The listing builds one solid part. Answer for the finished solid, in the listing's coordinates (mm). A direction names the side the tool comes from. Coordinates: 2 decimals unless noted, no trailing zeros. Order: outer loops, then holes, each group sorted by start corner. A loop starts at its lowest first (then second) coordinate and runs counter-clockwise, first axis right, second up. Notation, with made-up numbers: (3, 41) -> (41, 41) arc R24 cw to (41, 59) -> close; hole circle Ø2 at (12.5, 19.25). An arc over 180 degrees is marked (long way). Return JSON: item names as keys, results as strings.
```python
from build123d import *

# Parameters (mm, degrees)
SKETCH1_W           = 28
SKETCH1_H           = 5
BOSS_EXTRUDE1_DEPTH = 20
CHAMFER1_SIZE       = 15
BOSS_EXTRUDE2_DEPTH = 28
SKETCH3_W           = 3
SKETCH3_H           = 9
CUT_EXTRUDE1_DEPTH  = 12.8
CHAMFER2_SIZE       = 1
FILLET1_R           = 2
CHAMFER3_SIZE       = 0.5
CUT_EXTRUDE2_DEPTH  = 12.8
CHAMFER4_SIZE       = 3
CHAMFER5_SIZE       = 3
SKETCH8_W           = 3.20799886
SKETCH8_H           = 3.210000155
SKETCH8_W_2         = 3.209995615
SKETCH8_H_2         = 3.268000248
CUT_EXTRUDE3_DEPTH  = 5.4
SKETCH9_W           = 136.063633216
SKETCH9_H           = 34.178471192
CUT_EXTRUDE4_DEPTH  = 8
SKETCH10_W          = 4.648757297
SKETCH10_H          = 6.5
BOSS_EXTRUDE3_DEPTH = 10
SKETCH12_W          = 15
SKETCH12_H          = 15
BOSS_EXTRUDE4_DEPTH = 3
SKETCH13_R          = 1.5
CUT_EXTRUDE5_DEPTH  = 5
FILLET2_R           = 3
CHAMFER6_SIZE       = 3


with BuildPart() as part:
    # Sketch1 → Boss-Extrude1 (new body)
    with BuildSketch(Plane(origin=(0, 0, 0), x_dir=(1, 0, 0), z_dir=(0, 1, 0))):
        with Locations((14, 2.5)):
            Rectangle(SKETCH1_W, SKETCH1_H)
    extrude(amount=BOSS_EXTRUDE1_DEPTH)

    # Chamfer1
    chamfer1_edges = [part.edges().sort_by_distance(p)[0] for p in [
        (28, 0, -2.5),
    ]]
    chamfer(chamfer1_edges, length=CHAMFER1_SIZE)

    # Sketch2 → Boss-Extrude2 (add)
    with BuildSketch(Plane.XY):
        Polygon((9.648757297, 6.5), (5, 6.5), (5, 2), (5, 0), (9.648757297, 0), align=None)
    extrude(amount=BOSS_EXTRUDE2_DEPTH)

    # Sketch3 → Cut-Extrude1 (cut)
    with BuildSketch(Plane.XZ):
        with Locations((6.5, 18)):
            Rectangle(SKETCH3_W, SKETCH3_H)
    extrude(amount=-CUT_EXTRUDE1_DEPTH, mode=Mode.SUBTRACT)

    # Chamfer2
    chamfer2_edges = [part.edges().sort_by_distance(p)[0] for p in [
        (8, 3.25, 22.5),
        (8, 3.25, 13.5),
    ]]
    chamfer(chamfer2_edges, length=CHAMFER2_SIZE)

    # Fillet1
    fillet1_edges = [part.edges().sort_by_distance(p)[0] for p in [
        (7.324378649, 6.5, 28),
        (7.324378649, 0, 28),
    ]]
    fillet(fillet1_edges, radius=FILLET1_R)

    # Chamfer3
    chamfer3_edges = [part.edges().sort_by_distance(p)[0] for p in [
        (5, 3.25, 13.5),
        (5, 3.25, 22.5),
    ]]
    chamfer(chamfer3_edges, length=CHAMFER3_SIZE)

    # Sketch4 → Cut-Extrude2 (cut)
    with BuildSketch(Plane.ZY.offset(-5)):
        with BuildLine():
            ThreePointArc((25.5, 1.45), (27.05, 3), (25.5, 4.55))
            ThreePointArc((25.5, 4.55), (23.95, 3), (25.5, 1.45))
        make_face()
        with BuildLine():
            ThreePointArc((10.5, 4.55), (8.95, 3), (10.5, 1.45))
            ThreePointArc((10.5, 1.45), (12.05, 3), (10.5, 4.55))
        make_face()
    extrude(amount=-CUT_EXTRUDE2_DEPTH, mode=Mode.SUBTRACT)

    # Chamfer4
    chamfer4_edges = [part.edges().sort_by_distance(p)[0] for p in [
        (5, 3.25, 0),
        (9.648757297, 3.25, 0),
    ]]
    chamfer(chamfer4_edges, length=CHAMFER4_SIZE)

    # Chamfer5
    chamfer5_edges = [part.edges().sort_by_distance(p)[0] for p in [
        (7.324378649, 6.5, 0),
    ]]
    chamfer(chamfer5_edges, length=CHAMFER5_SIZE)

    # Sketch8 → Cut-Extrude3 (cut)
    # profile 1 of 4: a face of its own
    with BuildSketch(Plane(origin=(0, 20, 0), x_dir=(1, 0, 0), z_dir=(0, 1, 0))):
        with Locations((5.668003112, 2.226999903)):
            Rectangle(SKETCH8_W, SKETCH8_H)
        Polygon((7.122002542, 3.68199998), (6.328001618, 3.68199998), (4.214003682, 3.68199998), (4.214003682, 2.801999915), (4.214003682, 2.091999864), (4.214003682, 0.771999825), (4.858002067, 0.771999825), (6.60200417, 0.771999825), (7.122002542, 0.771999825), (7.122002542, 3.48399987), align=None, mode=Mode.SUBTRACT)
    # profile 2 of 4: a face of its own
    with BuildSketch(Plane(origin=(0, 20, 0), x_dir=(1, 0, 0), z_dir=(0, 1, 0))):
        Polygon((7.122002542, 3.68199998), (7.122002542, 3.48399987), (7.122002542, 0.771999825), (6.60200417, 0.771999825), (4.858002067, 0.771999825), (4.214003682, 0.771999825), (4.214003682, 2.091999864), (4.214003682, 2.801999915), (4.214003682, 3.68199998), (6.328001618, 3.68199998), align=None)
    # profile 3 of 4: a face of its own
    with BuildSketch(Plane(origin=(0, 20, 0), x_dir=(1, 0, 0), z_dir=(0, 1, 0))):
        with Locations((23.709002883, 2.229999751)):
            Rectangle(SKETCH8_W_2, SKETCH8_H_2)
        Polygon((22.254005075, 1.15799997), (22.254005075, 1.283999765), (22.254005075, 3.713999875), (25.16400069, 3.713999875), (25.16400069, 0.749999657), (25.16400069, 0.745999627), (24.429999292, 0.745999627), (22.254005075, 0.745999627), align=None, mode=Mode.SUBTRACT)
    # profile 4 of 4: a face of its own
    with BuildSketch(Plane(origin=(0, 20, 0), x_dir=(1, 0, 0), z_dir=(0, 1, 0))):
        Polygon((22.254005075, 3.713999875), (22.254005075, 1.283999765), (22.254005075, 1.15799997), (22.254005075, 0.745999627), (24.429999292, 0.745999627), (25.16400069, 0.745999627), (25.16400069, 0.749999657), (25.16400069, 3.713999875), align=None)
    extrude(amount=-CUT_EXTRUDE3_DEPTH, mode=Mode.SUBTRACT)

    # Sketch9 → Cut-Extrude4 (cut)
    with BuildSketch(Plane(origin=(0, 0, -5), x_dir=(-1, 0, 0), z_dir=(0, 0, -1))):
        with Locations((-4.69867378, 12.292617934)):
            Rectangle(SKETCH9_W, SKETCH9_H)
    extrude(amount=-CUT_EXTRUDE4_DEPTH, mode=Mode.SUBTRACT)

    # Sketch10 → Boss-Extrude3 (add)
    with BuildSketch(Plane(origin=(0, 0, 3), x_dir=(-1, 0, 0), z_dir=(0, 0, -1))):
        with Locations((-7.324378649, 3.25)):
            Rectangle(SKETCH10_W, SKETCH10_H)
    extrude(amount=BOSS_EXTRUDE3_DEPTH)

    # Sketch12 → Boss-Extrude4 (add)
    with BuildSketch(Plane(origin=(0, 0, -7), x_dir=(-1, 0, 0), z_dir=(0, 0, -1))):
        with Locations((-12.5, 7.5)):
            Rectangle(SKETCH12_W, SKETCH12_H)
    extrude(amount=-BOSS_EXTRUDE4_DEPTH)

    # Sketch13 → Cut-Extrude5 (cut)
    with BuildSketch(Plane.XY.offset(-4)):
        with Locations((17, 3)):
            Circle(SKETCH13_R)
        with Locations((8, 12)):
            Circle(SKETCH13_R)
    extrude(amount=-CUT_EXTRUDE5_DEPTH, mode=Mode.SUBTRACT)

    # Fillet2
    fillet2_edges = [part.edges().sort_by_distance(p)[0] for p in [
        (5, 15, -5.5),
        (20, 0, -5.5),
        (20, 15, -5.5),
    ]]
    fillet(fillet2_edges, radius=FILLET2_R)

    # Chamfer6
    chamfer6_edges = [part.edges().sort_by_distance(p)[0] for p in [
        (9.648757297, 3.25, -4),
    ]]
    chamfer(chamfer6_edges, length=CHAMFER6_SIZE)


solid = part.part
```
Item 1: The part is cut by section A-A on z = 25.5. Determine the outline of the cut face in (x, y).
Answer list:
{"outline": "(5, 0) -> (9.65, 0) -> (9.65, 1.45) -> (5, 1.45) -> close; (5, 4.55) -> (9.65, 4.55) -> (9.65, 6.5) -> (5, 6.5) -> close"}
Item 2: The part is cut by section B-B on y = 3.5. Determine the outline of the cut face in (x, z).
Answer list:
{"outline": "(5, -7) -> (15.59, -7) -> (15.59, -4) -> (12.65, -4) -> (9.65, -1) -> (9.65, 9.03) -> (5, 9.03) -> close; (5, 11.97) -> (9.65, 11.97) -> (9.65, 24.03) -> (5, 24.03) -> (5, 23) -> (5.5, 22.5) -> (7, 22.5) -> (8, 21.5) -> (8, 14.5) -> (7, 13.5) -> (5.5, 13.5) -> (5, 13) -> close; (5, 26.97) -> (9.65, 26.97) -> (9.65, 28) -> (5, 28) -> close; (18.41, -7) -> (20, -7) -> (20, -4) -> (18.41, -4) -> close"}
Item 3: The part is cut by section D-D on y = 13. Determine the outline of the cut face in (x, z).
Answer list:
{"outline": "(5.17, -7) -> (6.88, -7) -> (6.88, -4) -> (5.17, -4) -> close; (9.12, -7) -> (19.83, -7) -> (19.83, -4) -> (9.12, -4) -> close"}
Item 4: Which of the six approach directions +Z, -Z, +X, -X, +Y, -Y give full straight-line access (tool end or side, diameter ignored) to faces 4 (the flat face through (9.649, 3, 14)), 5 (the flat face through (6, 3, 22.5)), 6 (the cylindrical face through (6.8, 11.1, -5.5))?
Answer list:
{"face 4": "+Z, +X, +Y, -Y", "face 5": "-X, +Y, -Y", "face 6": "+Z, -Z"}
Item 5: Flat-ended cylindrical pins translate along their axes: pin 1 (5 mm diameter, centred on x = 13, y = 4.5, fed in from +Z); pin 2 (5 mm diameter, centred on y = 3, z = 25.5, fed in from +X); pin 3 (3 mm diameter, centred on x = 15, y = 10.5, fed in from +Z). Find the tip coordinate at first contact, or state that the pin passes through.
Answer list:
{"pin 1": "z = -1.85", "pin 2": "x = 9.65", "pin 3": "z = -4"}
Item 6: Find the intervals of material crossed by probe 1 along Z at (x, y) = (8.35, 3); probe 2 along Y at (x, z) = (17, -4.85); probe 3 along Y at (x, z) = (8.15, 25.5), in increasing order.
Answer list:
{"probe 1": "-7 to 8.95, 12.05 to 23.95, 27.05 to 28", "probe 2": "0 to 1.5, 4.5 to 15", "probe 3": "0 to 1.45, 4.55 to 6.5"}
Item 7: Determine the mould class of faces 1 (the flat face through (5, 3, 1)), 2 (the cylindrical face through (15.5, 3.07, -5.48)), 3 (the flat face through (7, 6.5, 8)) for opening direction Y: pulls with the +Y half, pulls with the -Y half, needs draft (parallel to the pull), parting line crosses it, or undercut.
Answer list:
{"face 1": "needs draft", "face 2": "undercut", "face 3": "pulls with the +Y half"}
Item 8: The part is cut by section C-C on x = 7.5. Determine the outline of the cut face in (y, z), plus the area to 3 significant figures.
Answer list:
{"outline": "(0, -7) -> (10.59, -7) -> (10.59, -4) -> (6.5, -4) -> (6.5, 14) -> (0, 14) -> close; (0, 22) -> (6.5, 22) -> (6.5, 26) arc R2 ccw to (4.5, 28) -> (2, 28) arc R2 ccw to (0, 26) -> close; (13.41, -7) -> (14.96, -7) -> (14.96, -4) -> (13.41, -4) -> close; hole circle Ø3.1 at (3, 10.5); hole circle Ø3.1 at (3, 25.5)", "area": "176 mm2"}
